Could you check a few things on this model? Use its own coordinates, in mm. Face numbers are marked on the shaded views. A direction names the side the tool comes from. Give positions to 0.01 mm unless a question says otherwise; leave off trailing zeros. Loops run counter-clockwise (first coordinate to the right, second up) from the corner with the lowest first, then second, coordinate; pieces in that order, holes last. Notation, with made-up numbers: M 71.25,59.5 L 110.25,59.5 A26 cw 110.25,98.5 Z; hole C 47.5,5.5 d5. An arc over 180 degrees is marked long. Use CSV: the item, a comma, the result in double quotes.
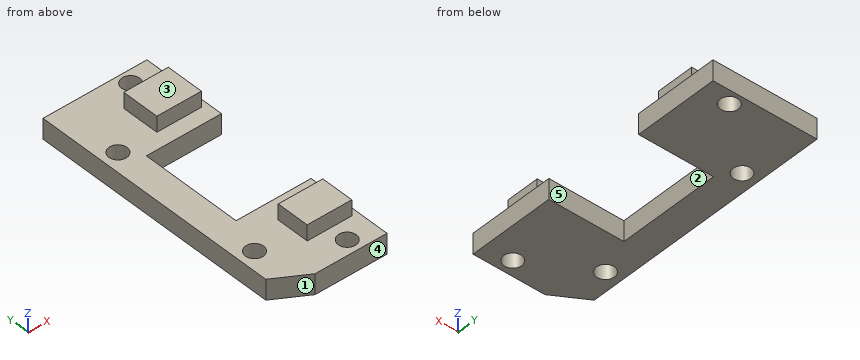
```python
from build123d import *

# Parameters (mm, degrees)
USB_END_CROSSBAR_WITH_OPEN_CONNECTOR_2_R       = 1.15
USB_END_CROSSBAR_WITH_OPEN_CONNECTOR_REL_DEPTH = 2.6
TWO_START                                      = 2.6
TWO_PCB_RESTS_BESIDE_TYPE_C_NO_SUPP_2_W        = 5.7
TWO_PCB_RESTS_BESIDE_TYPE_C_NO_SUPP_2_H        = 4.2
TWO_PCB_RESTS_BESIDE_TYPE_C_NO_SUPP_2_H_2      = 4.8
TWO_PCB_RESTS_BESIDE_TYPE_C_NO_SUPPORT_DEPTH   = 2


with BuildPart() as part:
    # USB end crossbar with open connector 2 → USB end crossbar with open connector rel (new body)
    with BuildSketch(Plane.XY):
        Polygon((-38.8, -21.5), (-34.7, -24), (-25.5, -24), (-25.5, -13), (-35.1, -13), (-35.1, 0), (-25.5, 0), (-25.5, 10.8), (-38.8, 10.8), align=None)
        with Locations((-36.8, -17.6)):
            Circle(USB_END_CROSSBAR_WITH_OPEN_CONNECTOR_2_R, mode=Mode.SUBTRACT)
        with Locations((-36.8, 2.2)):
            Circle(USB_END_CROSSBAR_WITH_OPEN_CONNECTOR_2_R, mode=Mode.SUBTRACT)
        with Locations((-29, -22.2)):
            Circle(USB_END_CROSSBAR_WITH_OPEN_CONNECTOR_2_R, mode=Mode.SUBTRACT)
        with Locations((-29, 9.2)):
            Circle(USB_END_CROSSBAR_WITH_OPEN_CONNECTOR_2_R, mode=Mode.SUBTRACT)
    extrude(amount=USB_END_CROSSBAR_WITH_OPEN_CONNECTOR_REL_DEPTH)

    # Two PCB rests beside Type-C_ no supp 2 → Two PCB rests beside Type-C_ no support (add)
    with BuildSketch(Plane.XY.offset(TWO_START)):
        with Locations((-29.15, -17.7)):
            Rectangle(TWO_PCB_RESTS_BESIDE_TYPE_C_NO_SUPP_2_W, TWO_PCB_RESTS_BESIDE_TYPE_C_NO_SUPP_2_H)
        with Locations((-29.15, 4.4)):
            Rectangle(TWO_PCB_RESTS_BESIDE_TYPE_C_NO_SUPP_2_W, TWO_PCB_RESTS_BESIDE_TYPE_C_NO_SUPP_2_H_2)
    extrude(amount=TWO_PCB_RESTS_BESIDE_TYPE_C_NO_SUPPORT_DEPTH)


solid = part.part
```
1. Please list where these lines run through material, in increasing order: line 1 (Y direction, x = -29, z = 1.4); line 2 (Y direction, x = -26.5, z = 1.85); line 3 (Y direction, x = -29.25, z = 4.35).
Outcome:
line 1,"-24 to -23.35, -21.05 to -13, 0 to 8.05, 10.35 to 10.8"
line 2,"-24 to -13, 0 to 10.8"
line 3,"-19.8 to -15.6, 2 to 6.8"
2. If we mould it in two halves opening along Y, with no side actions, what happens to the marked faces 3, 4 and 5? For each: +Y half, -Y half, draft (parallel to the pull), parting line (faces both ways), or undercut.
Outcome:
face 3,"draft"
face 4,"-Y half"
face 5,"undercut"
3. I want a section at A-A, the plane z = 3.55. List the corners of the cut face in (x, y) for me, then the cut area to 3 significant figures.
Outcome:
outline,"M -32,-19.8 L -26.3,-19.8 L -26.3,-15.6 L -32,-15.6 Z; M -32,2 L -26.3,2 L -26.3,6.8 L -32,6.8 Z"
area,"51.3 mm2"
4. I want a section at D-D, the plane z = 0.7. List the corners of the cut face in (x, y) for me, then the cut area to 3 significant figures.
Outcome:
outline,"M -38.8,-21.5 L -34.7,-24 L -25.5,-24 L -25.5,-13 L -35.1,-13 L -35.1,0 L -25.5,0 L -25.5,10.8 L -38.8,10.8 Z; hole C -36.8,-17.6 d2.3; hole C -36.8,2.2 d2.3; hole C -29,-22.2 d2.3; hole C -29,9.2 d2.3"
area,"316 mm2"
5. I want a section at C-C, the plane x = -30.75. List the corners of the cut face in (y, z) for me.
Outcome:
outline,"M -24,0 L -13,0 L -13,2.6 L -15.6,2.6 L -15.6,4.6 L -19.8,4.6 L -19.8,2.6 L -24,2.6 Z; M 0,0 L 10.8,0 L 10.8,2.6 L 6.8,2.6 L 6.8,4.6 L 2,4.6 L 2,2.6 L 0,2.6 Z"
6. I'm going to push flat-ended pins straight in: pin 1 Ø1.4 at (x, y) = (-36.8, -17.6) entering from -Z; pin 2 Ø0.6 at (y, z) = (-18, 3.5) entering from +X; pin 3 Ø0.6 at (x, z) = (-29, 4) entering from +Y; pin 4 Ø6.5 at (x, y) = (-35, 0.5) entering from +Z. Where does each tip first touch, or does it pass through?
Outcome:
pin 1,"through"
pin 2,"x = -26.3"
pin 3,"y = 6.8"
pin 4,"z = 2.6"
7. Which directions (+Z, -Z, +X, -X, +Y, -Y) give clear straight access to the entire face, cutting with the end or side of a thin tool? Please do the marked faces 1 and 2.
Outcome:
face 1,"+Z, -Z, -X, -Y"
face 2,"+Z, -Z, +X"
8. I want a section at B-B, the plane y = -17.6. List the corners of the cut face in (x, z) for me, then the cut area to 3 significant figures.
Outcome:
outline,"M -38.8,0 L -37.95,0 L -37.95,2.6 L -38.8,2.6 Z; M -35.65,0 L -25.5,0 L -25.5,2.6 L -26.3,2.6 L -26.3,4.6 L -32,4.6 L -32,2.6 L -35.65,2.6 Z"
area,"40.0 mm2"
